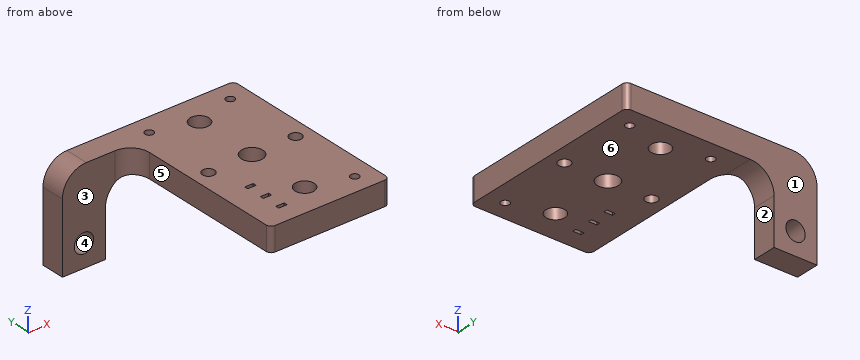
from build123d import *

# Parameters (mm, degrees)
ESBO_O1_W                     = 50
ESBO_O1_H                     = 80
RESSALTO_EXTRUS_O1_DEPTH      = 5
ESBO_O2_R                     = 4.5
ESBO_O2_R_2                   = 4
ESBO_O2_R_3                   = 2.5
CORTE_EXTRUS_O1_DEPTH         = 10
ESBO_O3_W                     = 3.5
ESBO_O3_H                     = 1.5
CORTE_EXTRUS_O2_DEPTH         = 22
ESBO_O4_R                     = 1.75
CORTE_EXTRUS_O3_DEPTH         = 10
FILETE1_R                     = 2
ESBO_O6_W                     = 30
ESBO_O6_H                     = 10
RESSALTO_EXTRUS_O2_DEPTH      = 29.5
RESSALTO_EXTRUS_O2_DEPTH_BACK = 10
ESBO_O7_R                     = 4.05
CORTE_EXTRUS_O4_DEPTH         = 50
ESBO_O8_W                     = 12
ESBO_O8_H                     = 29.5
CORTE_EXTRUS_O5_DEPTH         = 50
FILETE2_R                     = 10
FILETE3_R                     = 8


with BuildPart() as part:
    # Esboço1 → Ressalto-extrusão1 (new body, symmetric)
    with BuildSketch(Plane.XY):
        Rectangle(ESBO_O1_W, ESBO_O1_H)
    extrude(amount=RESSALTO_EXTRUS_O1_DEPTH, both=True)

    # Esboço2 → Corte-extrusão1 (cut)
    with BuildSketch(Plane.XY.offset(5)):
        Circle(ESBO_O2_R)
        with Locations((0, 27)):
            Circle(ESBO_O2_R_2)
        with Locations((0, -27)):
            Circle(ESBO_O2_R_2)
        with Locations((18.25, 0)):
            Circle(ESBO_O2_R_3)
        with Locations((-18.25, 0)):
            Circle(ESBO_O2_R_3)
    extrude(amount=-CORTE_EXTRUS_O1_DEPTH, mode=Mode.SUBTRACT)

    # Esboço3 → Corte-extrusão2 (cut)
    with BuildSketch(Plane.XY.offset(5)):
        with Locations((-13.25, -31.39)):
            Rectangle(ESBO_O3_W, ESBO_O3_H)
        with Locations((-13.25, -23.39)):
            Rectangle(ESBO_O3_W, ESBO_O3_H)
        with Locations((-13.25, -15.39)):
            Rectangle(ESBO_O3_W, ESBO_O3_H)
    extrude(amount=-CORTE_EXTRUS_O2_DEPTH, mode=Mode.SUBTRACT)

    # Esboço4 → Corte-extrusão3 (cut)
    with BuildSketch(Plane.XY.offset(5)):
        with Locations((-17, 32)):
            Circle(ESBO_O4_R)
        with Locations((17, 32)):
            Circle(ESBO_O4_R)
        with Locations((17, -32)):
            Circle(ESBO_O4_R)
    extrude(amount=-CORTE_EXTRUS_O3_DEPTH, mode=Mode.SUBTRACT)

    # Filete1
    filete1_edges = [part.edges().sort_by_distance(p)[0] for p in [
        (25, -40, 0),
        (-25, -40, 0),
        (25, 40, 0),
    ]]
    fillet(filete1_edges, radius=FILETE1_R)

    # Esboço6 → Ressalto-extrusão2 (add, two sides)
    with BuildSketch(Plane(origin=(0, 0, -5), x_dir=(-1, 0, 0), z_dir=(0, 0, -1))) as ressalto_extrus_o2_sk:
        with Locations((40, 35)):
            Rectangle(ESBO_O6_W, ESBO_O6_H)
    extrude(amount=RESSALTO_EXTRUS_O2_DEPTH)
    extrude(ressalto_extrus_o2_sk.sketch, amount=-RESSALTO_EXTRUS_O2_DEPTH_BACK)

    # Esboço7 → Corte-extrusão4 (cut)
    with BuildSketch(Plane(origin=(0, 40, 0), x_dir=(1, 0, 0), z_dir=(0, 1, 0))):
        with Locations((-46, 25)):
            Circle(ESBO_O7_R)
    extrude(amount=-CORTE_EXTRUS_O4_DEPTH, mode=Mode.SUBTRACT)

    # Esboço8 → Corte-extrusão5 (cut)
    with BuildSketch(Plane(origin=(0, 40, 0), x_dir=(1, 0, 0), z_dir=(0, 1, 0))):
        with Locations((-31, 19.75)):
            Rectangle(ESBO_O8_W, ESBO_O8_H)
    extrude(amount=-CORTE_EXTRUS_O5_DEPTH, mode=Mode.SUBTRACT)

    # Filete2
    filete2_edges = [part.edges().sort_by_distance(p)[0] for p in [
        (-55, 35, 5),
        (-37, 35, -5),
    ]]
    fillet(filete2_edges, radius=FILETE2_R)

    # Filete3
    filete3_edges = [part.edges().sort_by_distance(p)[0] for p in [
        (-25, 30, 0),
    ]]
    fillet(filete3_edges, radius=FILETE3_R)


solid = part.part
The listing builds one solid part. Answer for the finished solid, in the listing's coordinates (mm). Face numbers are marked on the shaded views. A direction names the side the tool comes from. Round coordinates to 2 decimals unless told otherwise and drop trailing zeros. Order: outer loops, then holes, each group sorted by start corner. A loop starts at its lowest first (then second) coordinate and runs counter-clockwise, first axis right, second up. Notation, with made-up numbers: (30, 32.5) - (46, 32.5) arc R21 ccw to (46, 67.5) - close; hole circle Ø6 at (68.25, 60.25). An arc over 180 degrees is marked (long way). Write item = value, one per line. Start each with the question number.
1) Given pin 1 (5.5 mm diameter, centred on x = 0, y = 0, fed in from -Z); pin 2 (8 mm diameter, centred on x = -18.25, y = 0, fed in from -Z); pin 3 (8 mm diameter, centred on y = 3.5, z = -6, fed in from -X); pin 4 (3 mm diameter, centred on x = -38, z = -21.5, fed in from -Y), each flat-ended and moving along its own axis, determine where each tip first touches the part or whether it passes through.
2) Straight lines are drawn through the part: L1, parallel to Y at x = 0, z = 2; L2, parallel to Y at x = 18, z = -1; L3, parallel to Z at x = -13, y = -17. For each, find the intervals that lie inside material, in ascending order.
3) Section B-B, the plane z = -25 is taken. Write down the section's boundary in (x, y).
4) For a pull along X with two mould halves and no side action, classify the marked faces 4, 5 and 6 as released by +X, released by -X, zero draft, split by the parting line, or undercut.
5) Section C-C, the plane x = 0 is taken. Write down the section's boundary in (y, z), plus the area to 3 significant figures.
6) For the marked faces 1, 2 and 3, determine the directions among +Z, -Z, +X, -X, +Y, -Y from which every point of the face is accessible in a straight line to the end or side of a thin tool.
7) Section D-D, the plane y = 0 is taken. Write down the section's boundary in (x, z), plus the area to 3 significant figures.
8) Section A-A, the plane y = 32 is taken. Write down the section's boundary in (x, z), plus the area to 3 significant figures.
Results list:
q1.pin_1 = through
q1.pin_2 = -5
q1.pin_3 = -25
q1.pin_4 = 30
q2.L1 = -40 to -31, -23 to -4.5, 4.5 to 23, 31 to 40
q2.L2 = -40 to -33.44, -30.56 to -2.49, 2.49 to 30.56, 33.44 to 40
q2.L3 = -5 to 5
q3.outline = (-55, 30) - (-50.05, 30) - (-50.05, 40) - (-55, 40) - close; (-41.95, 30) - (-37, 30) - (-37, 40) - (-41.95, 40) - close
q4.face_4 = undercut
q4.face_5 = released by -X
q4.face_6 = zero draft
q5.outline = (-40, -5) - (-31, -5) - (-31, 5) - (-40, 5) - close; (-23, -5) - (-4.5, -5) - (-4.5, 5) - (-23, 5) - close; (4.5, -5) - (23, -5) - (23, 5) - (4.5, 5) - close; (31, -5) - (40, -5) - (40, 5) - (31, 5) - close
q5.area = 550 mm^2
q6.face_1 = +Z, -Z, +X, -X, +Y
q6.face_2 = -Z, +X, +Y, -Y
q6.face_3 = +Z, -Z, -X, -Y
q7.outline = (-25, -5) - (-20.75, -5) - (-20.75, 5) - (-25, 5) - close; (-15.75, -5) - (-4.5, -5) - (-4.5, 5) - (-15.75, 5) - close; (4.5, -5) - (15.75, -5) - (15.75, 5) - (4.5, 5) - close; (20.75, -5) - (25, -5) - (25, 5) - (20.75, 5) - close
q7.area = 310 mm^2
q8.outline = (-55, -34.5) - (-37, -34.5) - (-37, -15) arc R10 cw to (-27, -5) - (-18.75, -5) - (-18.75, 5) - (-45, 5) arc R10 ccw to (-55, -5) - close; (-15.25, -5) - (15.25, -5) - (15.25, 5) - (-15.25, 5) - close; (18.75, -5) - (25, -5) - (25, 5) - (18.75, 5) - close; hole circle Ø8.1 at (-46, -25)
q8.area = 1,210 mm^2
